Geometry: final body of the model. Coordinates: model frame, mm. A direction names the side the tool comes from. Coordinates: 2 decimals unless noted, no trailing zeros. Order: outer loops, then holes, each group sorted by start corner. A loop starts at its lowest first (then second) coordinate and runs counter-clockwise, first axis right, second up. Notation, with made-up numbers: (88, 12.5) - (144, 12.5) arc R26 ccw to (144, 48.5) - close; hole circle Ø10 at (3, 23). An arc over 180 degrees is marked (long way). Use a Markdown table: item, result. Add a question column.
```python
from build123d import *

# Parameters (mm, degrees)
F2_SIZE  = 0.5
F3_R     = 0.5
F6_DEPTH = 3.5


with BuildPart() as f1:
    # F0 (on Front) → F1 (revolve)
    with BuildSketch(Plane.XZ):
        Polygon((0, 15), (0, 0), (0, -42), (2.5, -44.5), (2.5, -47), (15, -47), (15, -45), (15, -42), (12.5, -42), (12.5, -30), (11.95, -30), (11.95, -28.7), (12.475, -28.7), (12.475, -24), (7, -24), (7, 16), (6.7, 16), (6.7, 17.1), (6.975, 17.1), (6.975, 20), (2.5, 20), (2.5, 17.5), align=None)
    revolve(axis=Axis((0, 0, 55.465363), (0, 0, 1)))

    # F2
    f2_edges = [f1.edges().sort_by_distance(p)[0] for p in [
        (-6.975, 0, 20),
        (-12.475, 0, -24),
        (-7, 0, -24),
        (-15, 0, -42),
    ]]
    chamfer(f2_edges, length=F2_SIZE)

    # F3
    f3_edges = [f1.edges().sort_by_distance(p)[0] for p in [
        (-12.5, 0, -42),
    ]]
    fillet(f3_edges, radius=F3_R)

    # F5 (on offset) → F6 (cut)
    with BuildSketch(Plane.XZ.offset(7)):
        with BuildLine():
            Line((3, -18.5), (3, 10.5))
            ThreePointArc((3, 10.5), (0, 13.5), (-3, 10.5))
            Line((-3, 10.5), (-3, -18.5))
            ThreePointArc((-3, -18.5), (0, -21.5), (3, -18.5))
        make_face()
    extrude(amount=-F6_DEPTH, mode=Mode.SUBTRACT)


solid = f1.part
```
1) Set-up query: faces 4 (the face through (3.763, 5.902, -3.473)), 5 (the face through (6.42, 10.08, -29.34)), 6 (the face through (3, -5, -4)). Return all of +Z, -Z, +X, -X, +Y, -Y with unobstructed straight access to the full face (end or side cutting, diameter ignored); none if empty.
2) Section B-B (z = -16.5). Return loops of the section in (x, y).
3) Pin query (flat end, axial travel): pin 1 (6 mm diameter, centred on y = 3.5, z = -29.5, fed in from +X); pin 2 (3 mm diameter, centred on x = -1, z = 2, fed in from -Y); pin 3 (6 mm diameter, centred on x = 0, y = 0, fed in from -Z); pin 4 (4 mm diameter, centred on x = 7, z = -39.5, fed in from +Y). Return the tip coordinate at first contact, or that it passes through.
4) Section C-C (z = 12). Return loops of the section in (x, y).
5) Ray query, line 1 along Y through (x, z) = (0, 18.5) (3 decimals); line 2 along Y through (x, z) = (0, -45.4); line 3 along Y through (x, z) = (-0.5, -37.5). Return the intervals inside material, ascending.
6) Section A-A (z = -33). Return loops of the section in (x, y), then the cut area to 3 significant figures.
7) Draft query along Y for faces 1 (the face through (-0.54, -2.44, 18.73)), 2 (the face through (11.923, 3.755, -35.669)), 3 (the face through (-3, -5, -4)). Return one class per face: pulls with the +Y half, pulls with the -Y half, needs draft (parallel to the pull), parting line crosses it, or undercut.
Values follow:
| question | item | result |
|---|---|---|
| 1 | face 4 | +Z |
| 1 | face 5 | none |
| 1 | face 6 | -Y |
| 2 | outline | (-3, -6.32) - (-3, -3.5) - (3, -3.5) - (3, -6.32) arc R7 ccw (long way) to start |
| 3 | pin 1 | stops at x = 12.49 |
| 3 | pin 2 | stops at y = -3.5 |
| 3 | pin 3 | stops at z = -47 |
| 3 | pin 4 | stops at y = 11.46 |
| 4 | outline | (-2.6, -6.5) - (-2.6, -3.5) - (2.6, -3.5) - (2.6, -6.5) arc R7 ccw (long way) to start |
| 5 | line 1 | y = -6.975 to -2.5, 2.5 to 6.975 |
| 5 | line 2 | y = -15 to -2.5, 2.5 to 15 |
| 5 | line 3 | y = -12.49 to 12.49 |
| 6 | outline | circle Ø25 at (0, 0) |
| 6 | area | 491 mm² |
| 7 | face 1 | undercut |
| 7 | face 2 | parting line crosses it |
| 7 | face 3 | needs draft |
